```python
from build123d import *

# Parameters (mm, degrees)
SKETCH1_R           = 1.6
BOSS_EXTRUDE1_DEPTH = 2.8
FILLET1_R           = 3


with BuildPart() as part:
    # Sketch1 → Boss-Extrude1 (new body)
    with BuildSketch(Plane.XY):
        Polygon((-20, 20), (20, 20), (20, -20), (-20, -20), (-20, -9.55), (-12.5, -9.55), (-12.5, 2.95), (-20, 2.95), align=None)
        with Locations((-16, 16)):
            Circle(SKETCH1_R, mode=Mode.SUBTRACT)
        with Locations((16, 16)):
            Circle(SKETCH1_R, mode=Mode.SUBTRACT)
        with Locations((16, -16)):
            Circle(SKETCH1_R, mode=Mode.SUBTRACT)
        with Locations((-16, -16)):
            Circle(SKETCH1_R, mode=Mode.SUBTRACT)
    extrude(amount=BOSS_EXTRUDE1_DEPTH)

    # Fillet1
    fillet1_edges = [part.edges().sort_by_distance(p)[0] for p in [
        (20, -20, 1.4),
        (-20, -20, 1.4),
        (-20, -9.55, 1.4),
        (-20, 2.95, 1.4),
        (-20, 20, 1.4),
        (20, 20, 1.4),
    ]]
    fillet(fillet1_edges, radius=FILLET1_R)


solid = part.part
```
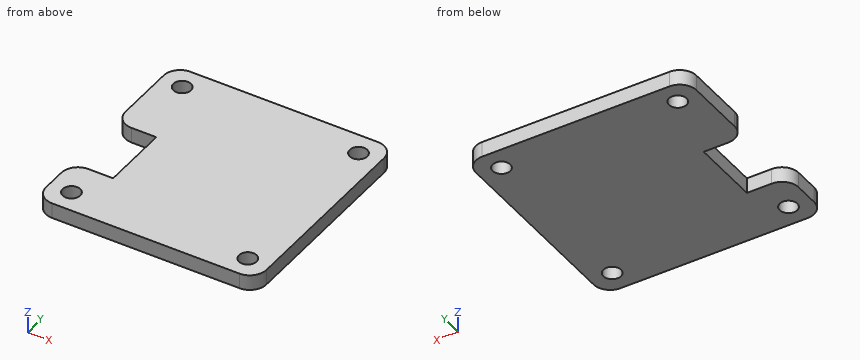
Here's how the part is built. I have some questions about the finished solid (model axes, mm). Give positions to 0.01 mm unless a question says otherwise; leave off trailing zeros. Write each loop counter-clockwise with the first axis right and the second up, starting at its lowest first coordinate (ties: lowest second). Pieces come first, ordered by that corner, then holes.
(1) Will this pin go through, and if not, where does the flat tip stop? pin 1 (0.8 mm diameter, centred on y = -2.5, z = 1.5, fed in from -X).
Output values:
pin 1: stops at x = -12.5
(2) Imagine slicing it at C-C, the plane x = -16. Write out the boundary of the cut face in (y, z).
Output values:
outline: (-20, 0) - (-17.6, 0) - (-17.6, 2.8) - (-20, 2.8) - close; (-14.4, 0) - (-9.55, 0) - (-9.55, 2.8) - (-14.4, 2.8) - close; (2.95, 0) - (14.4, 0) - (14.4, 2.8) - (2.95, 2.8) - close; (17.6, 0) - (20, 0) - (20, 2.8) - (17.6, 2.8) - close
(3) Imagine slicing it at A-A, the plane x = 16. Write out the boundary of the cut face in (y, z).
Output values:
outline: (-20, 0) - (-17.6, 0) - (-17.6, 2.8) - (-20, 2.8) - close; (-14.4, 0) - (14.4, 0) - (14.4, 2.8) - (-14.4, 2.8) - close; (17.6, 0) - (20, 0) - (20, 2.8) - (17.6, 2.8) - close
(4) Imagine slicing it at D-D, the plane z = 0.7. Write out the boundary of the cut face in (x, y).
Output values:
outline: (-20, -17) arc R3 ccw to (-17, -20) - (17, -20) arc R3 ccw to (20, -17) - (20, 17) arc R3 ccw to (17, 20) - (-17, 20) arc R3 ccw to (-20, 17) - (-20, 5.95) arc R3 ccw to (-17, 2.95) - (-12.5, 2.95) - (-12.5, -9.55) - (-17, -9.55) arc R3 ccw to (-20, -12.55) - close; hole circle Ø3.2 at (-16, -16); hole circle Ø3.2 at (-16, 16); hole circle Ø3.2 at (16, -16); hole circle Ø3.2 at (16, 16)
(5) If I drill on L1, parallel to Y at x = 16, z = 1.2; L2, parallel to Y at x = -16, z = 1.65; L3, parallel to Y at x = -13, z = 2.6, over which ranges is the centre line in solid material (lowest first)?
Output values:
L1: y = -20 to -17.6, -14.4 to 14.4, 17.6 to 20
L2: y = -20 to -17.6, -14.4 to -9.55, 2.95 to 14.4, 17.6 to 20
L3: y = -20 to -9.55, 2.95 to 20
